Geometry check sheet. Reference: the model listing, model coordinates, mm. Round coordinates to 2 decimals unless told otherwise and drop trailing zeros. Loops run counter-clockwise (first coordinate to the right, second up) from the corner with the lowest first, then second, coordinate; pieces in that order, holes last. Notation, with made-up numbers: M -10.75,51 L 15.25,51 A22 cw 15.25,72 Z; hole C 8.25,2 d5. An arc over 180 degrees is marked long. Answer in a Markdown table with one row per item. Add a question column.
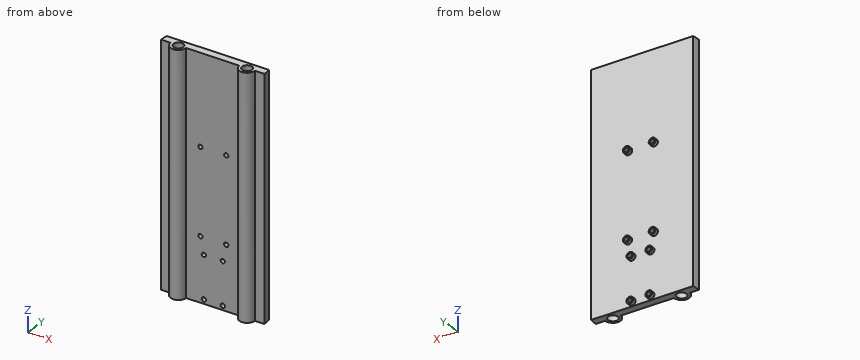
```python
from build123d import *

# Parameters (mm, degrees)
SKETCH1_R           = 5.715
SKETCH1_R_2         = 3.683
BOSS_EXTRUDE2_DEPTH = 177.8
SKETCH2_R           = 1.5875
CUT_EXTRUDE1_DEPTH  = 183.195210969
BOSS_EXTRUDE4_START = 2.54
SKETCH3_R           = 2.521654131
SKETCH3_R_2         = 1.5875
SKETCH3_R_3         = 2.580622747
SKETCH3_R_4         = 2.513629008
SKETCH3_R_5         = 2.53806637
BOSS_EXTRUDE4_DEPTH = 2.54
SKETCH4_R           = 1.5875
CUT_EXTRUDE2_DEPTH  = 183.195210969
BOSS_EXTRUDE5_START = 2.54
SKETCH5_R           = 2.618871397
SKETCH5_R_2         = 1.5875
SKETCH5_R_3         = 2.639509757
SKETCH5_R_4         = 2.648115463
SKETCH5_R_5         = 2.550190152
BOSS_EXTRUDE5_DEPTH = 2.54


with BuildPart() as part:
    # Sketch1 → Boss-Extrude2 (new body)
    # profile 1 of 5: a face of its own
    with BuildSketch(Plane.XY):
        with BuildLine():
            Line((25.4, 5.715), (-25.4, 5.715))
            ThreePointArc((-25.4, 5.715), (-21.358884746, 4.041115254), (-19.685, 0))
            Line((-19.685, 0), (19.685, 0))
            ThreePointArc((19.685, 0), (21.358884746, 4.041115254), (25.4, 5.715))
        make_face()
    # profile 2 of 5: a face of its own
    with BuildSketch(Plane.XY):
        with Locations((-25.4, 0)):
            Circle(SKETCH1_R)
        with Locations((-25.4, 0)):
            Circle(SKETCH1_R_2, mode=Mode.SUBTRACT)
    # profile 3 of 5: a face of its own
    with BuildSketch(Plane.XY):
        with Locations((25.4, 0)):
            Circle(SKETCH1_R)
        with Locations((25.4, 0)):
            Circle(SKETCH1_R_2, mode=Mode.SUBTRACT)
    # profile 4 of 5: a face of its own
    with BuildSketch(Plane.XY):
        with BuildLine():
            ThreePointArc((-31.115, 0), (-29.441115254, 4.041115254), (-25.4, 5.715))
            Line((-25.4, 5.715), (-37.668936473, 5.715))
            ThreePointArc((-37.668936473, 5.715), (-37.992081278, 2.865616895), (-38.1, 0))
            Line((-38.1, 0), (-31.115, 0))
        make_face()
    # profile 5 of 5: a face of its own
    with BuildSketch(Plane.XY):
        with BuildLine():
            Line((37.668936473, 5.715), (25.4, 5.715))
            ThreePointArc((25.4, 5.715), (29.441115254, 4.041115254), (31.115, 0))
            Line((31.115, 0), (38.1, 0))
            ThreePointArc((38.1, 0), (37.992081278, 2.865616895), (37.668936473, 5.715))
        make_face()
    extrude(amount=BOSS_EXTRUDE2_DEPTH)

    # Sketch2 → Cut-Extrude1 (cut, through all)
    with BuildSketch(Plane(origin=(0, 5.715, 0), x_dir=(1, 0, 0), z_dir=(0, 1, 0))):
        with Locations(Location((-6.553936473, -3.175, 0), (0, 0, 270))):
            Circle(SKETCH2_R)
        with Locations(Location((7.416063527, -3.175, 0), (0, 0, 270))):
            Circle(SKETCH2_R)
        with Locations(Location((-6.553936473, -34.925, 0), (0, 0, 270))):
            Circle(SKETCH2_R)
        with Locations(Location((7.416063527, -34.925, 0), (0, 0, 270))):
            Circle(SKETCH2_R)
    extrude(amount=-CUT_EXTRUDE1_DEPTH, mode=Mode.SUBTRACT)

    # Sketch3 → Boss-Extrude4 (add)
    # profile 1 of 4: a face of its own
    with BuildSketch(Plane(origin=(0, 5.715, 0), x_dir=(1, 0, 0), z_dir=(0, 1, 0)).offset(BOSS_EXTRUDE4_START)):
        with Locations(Location((-6.553936473, -3.175, 0), (0, 0, 270))):
            Circle(SKETCH3_R)
        with Locations(Location((-6.553936473, -3.175, 0), (0, 0, 270))):
            Circle(SKETCH3_R_2, mode=Mode.SUBTRACT)
    # profile 2 of 4: a face of its own
    with BuildSketch(Plane(origin=(0, 5.715, 0), x_dir=(1, 0, 0), z_dir=(0, 1, 0)).offset(BOSS_EXTRUDE4_START)):
        with Locations(Location((7.416063527, -3.175, 0), (0, 0, 270))):
            Circle(SKETCH3_R_3)
        with Locations(Location((7.416063527, -3.175, 0), (0, 0, 270))):
            Circle(SKETCH3_R_2, mode=Mode.SUBTRACT)
    # profile 3 of 4: a face of its own
    with BuildSketch(Plane(origin=(0, 5.715, 0), x_dir=(1, 0, 0), z_dir=(0, 1, 0)).offset(BOSS_EXTRUDE4_START)):
        with Locations(Location((7.416063527, -34.925, 0), (0, 0, 270))):
            Circle(SKETCH3_R_4)
        with Locations(Location((7.416063527, -34.925, 0), (0, 0, 270))):
            Circle(SKETCH3_R_2, mode=Mode.SUBTRACT)
    # profile 4 of 4: a face of its own
    with BuildSketch(Plane(origin=(0, 5.715, 0), x_dir=(1, 0, 0), z_dir=(0, 1, 0)).offset(BOSS_EXTRUDE4_START)):
        with Locations(Location((-6.553936473, -34.925, 0), (0, 0, 270))):
            Circle(SKETCH3_R_5)
        with Locations(Location((-6.553936473, -34.925, 0), (0, 0, 270))):
            Circle(SKETCH3_R_2, mode=Mode.SUBTRACT)
    extrude(amount=-BOSS_EXTRUDE4_DEPTH)

    # Sketch4 → Cut-Extrude2 (cut, through all)
    with BuildSketch(Plane(origin=(0, 5.715, 0), x_dir=(1, 0, 0), z_dir=(0, 1, 0))):
        with Locations(Location((-9.093936473, -47.368407893, 0), (0, 0, 270))):
            Circle(SKETCH4_R)
        with Locations(Location((9.956063527, -47.368407893, 0), (0, 0, 270))):
            Circle(SKETCH4_R)
        with Locations(Location((9.956063527, -110.868407893, 0), (0, 0, 270))):
            Circle(SKETCH4_R)
        with Locations(Location((-9.093936473, -110.868407893, 0), (0, 0, 270))):
            Circle(SKETCH4_R)
    extrude(amount=-CUT_EXTRUDE2_DEPTH, mode=Mode.SUBTRACT)

    # Sketch5 → Boss-Extrude5 (add)
    # profile 1 of 4: a face of its own
    with BuildSketch(Plane(origin=(0, 5.715, 0), x_dir=(1, 0, 0), z_dir=(0, 1, 0)).offset(BOSS_EXTRUDE5_START)):
        with Locations(Location((-9.093936473, -47.368407893, 0), (0, 0, 270))):
            Circle(SKETCH5_R)
        with Locations(Location((-9.093936473, -47.368407893, 0), (0, 0, 270))):
            Circle(SKETCH5_R_2, mode=Mode.SUBTRACT)
    # profile 2 of 4: a face of its own
    with BuildSketch(Plane(origin=(0, 5.715, 0), x_dir=(1, 0, 0), z_dir=(0, 1, 0)).offset(BOSS_EXTRUDE5_START)):
        with Locations(Location((9.956063527, -47.368407893, 0), (0, 0, 270))):
            Circle(SKETCH5_R_3)
        with Locations(Location((9.956063527, -47.368407893, 0), (0, 0, 270))):
            Circle(SKETCH5_R_2, mode=Mode.SUBTRACT)
    # profile 3 of 4: a face of its own
    with BuildSketch(Plane(origin=(0, 5.715, 0), x_dir=(1, 0, 0), z_dir=(0, 1, 0)).offset(BOSS_EXTRUDE5_START)):
        with Locations(Location((9.956063527, -110.868407893, 0), (0, 0, 270))):
            Circle(SKETCH5_R_4)
        with Locations(Location((9.956063527, -110.868407893, 0), (0, 0, 270))):
            Circle(SKETCH5_R_2, mode=Mode.SUBTRACT)
    # profile 4 of 4: a face of its own
    with BuildSketch(Plane(origin=(0, 5.715, 0), x_dir=(1, 0, 0), z_dir=(0, 1, 0)).offset(BOSS_EXTRUDE5_START)):
        with Locations(Location((-9.093936473, -110.868407893, 0), (0, 0, 270))):
            Circle(SKETCH5_R_5)
        with Locations(Location((-9.093936473, -110.868407893, 0), (0, 0, 270))):
            Circle(SKETCH5_R_2, mode=Mode.SUBTRACT)
    extrude(amount=-BOSS_EXTRUDE5_DEPTH)


solid = part.part
```
1) Cross-section at C-C, the plane y = -1.75. Record the boundary of the cut face in (x, z).
2) Cross-section at B-B, the plane x = -25.4. Record the boundary of the cut face in (y, z) (3 decimals), plus the area to 3 significant figures.
3) Thickness scan on L1, parallel to X at y = 1.5, z = 83.5; L2, parallel to X at y = -0.5, z = 59.5; L3, parallel to Z at x = 7.5, y = 3. Record the ranges inside material, lowest first. Write a range as [from, to].
4) Cross-section at A-A, the plane z = 119.5. Record the boundary of the cut face in (x, y) (3 decimals), plus the area to 3 significant figures.
5) Go/stop test with flat-tipped pins: pin 1 (1.5 mm diameter, centred on y = -2, z = 27.5, fed in from -X); pin 2 (5.5 mm diameter, centred on x = 36, z = 85, fed in from -Y); pin 3 (2 mm diameter, centred on y = -2.5, z = 77, fed in from +X); pin 4 (2.5 mm diameter, centred on x = 9.96, z = 110.87, fed in from +Y). Record where each tip stops, or that it passes through.
6) Cross-section at D-D, the plane x = 15.5. Record the boundary of the cut face in (y, z) (3 decimals), plus the area to 3 significant figures.
Worked answers:
| question | item | result |
|---|---|---|
| 1 | outline | M -30.84,0 L -28.64,0 L -28.64,177.8 L -30.84,177.8 Z; M -22.16,0 L -19.96,0 L -19.96,177.8 L -22.16,177.8 Z; M 19.96,0 L 22.16,0 L 22.16,177.8 L 19.96,177.8 Z; M 28.64,0 L 30.84,0 L 30.84,177.8 L 28.64,177.8 Z |
| 2 | outline | M -5.715,0 L -3.683,0 L -3.683,177.8 L -5.715,177.8 Z; M 3.683,0 L 5.715,0 L 5.715,177.8 L 3.683,177.8 Z |
| 2 | area | 723 mm2 |
| 3 | L1 | x = [-38.07, -28.76], [-22.04, 22.04], [28.76, 38.07] |
| 3 | L2 | x = [-31.09, -29.05], [-21.75, -19.71], [19.71, 21.75], [29.05, 31.09] |
| 3 | L3 | z = [0, 1.59], [4.76, 33.34], [36.51, 177.8] |
| 4 | outline | M -38.1,0 L -31.115,0 A5.715 ccw -19.685,0 L 19.685,0 A5.715 ccw 31.115,0 L 38.1,0 A38.1 ccw 37.669,5.715 L -37.669,5.715 A38.1 ccw Z; hole C -25.4,0 d7.366; hole C 25.4,0 d7.366 |
| 4 | area | 451 mm2 |
| 5 | pin 1 | stops at x = -30.98 |
| 5 | pin 2 | stops at y = 0 |
| 5 | pin 3 | stops at x = 30.91 |
| 5 | pin 4 | passes through |
| 6 | outline | M 0,0 L 5.715,0 L 5.715,177.8 L 0,177.8 Z |
| 6 | area | 1,020 mm2 |
